from build123d import *

# Parameters (mm, degrees)
SKETCH2_R           = 3.175
SKETCH2_R_2         = 2
SKETCH2_R_3         = 1.905
SKETCH2_R_4         = 1.999999991
BOSS_EXTRUDE1_DEPTH = 6.35
FILLET3_R           = 2.54
FILLET4_R           = 2.54
FILLET5_R           = 2.54


with BuildPart() as part:
    # Sketch2 → Boss-Extrude1 (new body)
    with BuildSketch(Plane(origin=(0, 0, 0), x_dir=(1, 0, 0), z_dir=(0, 1, 0))):
        with BuildLine():
            Line((13.846627418, -27.11715969), (17.295902343, -28.359470371))
            Line((17.295902343, -28.359470371), (17.295902343, -164.950770806))
            Line((17.295902343, -164.950770806), (-5.788689103, -224.106088723))
            Line((-5.788689103, -224.106088723), (-16.51, -231.775))
            Line((-16.51, -231.775), (-16.51, -118.11))
            Line((-16.51, -118.11), (-16.51, -40.527182032))
            Line((-16.51, -40.527182032), (-12.5603, 0))
            ThreePointArc((-12.5603, 0), (0, 12.5603), (12.5603, 0))
            Line((12.5603, 0), (11.834308479, -23.392641285))
            ThreePointArc((11.834308479, -23.392641285), (12.129138804, -25.639224299), (13.846627418, -27.11715969))
        make_face()
        with Locations(Location((0, 0, 0), (0, 0, 270))):
            Circle(SKETCH2_R, mode=Mode.SUBTRACT)
        with Locations(Location((-11.43, -219.075, 0), (0, 0, 270))):
            Circle(SKETCH2_R_2, mode=Mode.SUBTRACT)
        with Locations(Location((-11.43, -212.725, 0), (0, 0, 270))):
            Circle(SKETCH2_R_2, mode=Mode.SUBTRACT)
        with Locations(Location((-11.43, -206.375, 0), (0, 0, 270))):
            Circle(SKETCH2_R_2, mode=Mode.SUBTRACT)
        with Locations(Location((-11.43, -200.025, 0), (0, 0, 270))):
            Circle(SKETCH2_R_2, mode=Mode.SUBTRACT)
        with Locations(Location((-10.6553, -63.5, 0), (0, 0, 270))):
            Circle(SKETCH2_R_3, mode=Mode.SUBTRACT)
        with Locations(Location((13.485902343, -38.1, 0), (0, 0, 270))):
            Circle(SKETCH2_R_4, mode=Mode.SUBTRACT)
        Polygon((-3.088444979, -200.025), (-8.437091633, -150.367410486), (11.707902343, -162.914359455), align=None, mode=Mode.SUBTRACT)
        Polygon((5.669829362, -152.570430441), (11.707902343, -156.331136136), (11.707902343, -148.173239335), align=None, mode=Mode.SUBTRACT)
        Polygon((-9.197164207, -143.310789567), (1.48362655, -149.963128939), (11.707902343, -142.517360277), (11.707902343, -83.82613362), (-6.752611098, -71.345410911), (-11.894481361, -75.089947663), (-11.894481361, -118.268516882), align=None, mode=Mode.SUBTRACT)
        with BuildLine():
            Line((-5.45038708, -57.047318199), (5.477174601, -46.119756518))
            Line((5.477174601, -46.119756518), (9.770631453, -46.119756518))
            Line((9.770631453, -46.119756518), (11.707902343, -77.037423395))
            Line((11.707902343, -77.037423395), (-4.240626345, -66.254995008))
            ThreePointArc((-4.240626345, -66.254995008), (-4.111536449, -61.554723114), (-5.45038708, -57.047318199))
        make_face(mode=Mode.SUBTRACT)
        Polygon((-10.6553, -40.527182032), (-8.00152211, -13.297230483), (5.477174601, -13.297230483), (5.477174601, -31.974105906), (1.94113758, -40.527182032), align=None, mode=Mode.SUBTRACT)
        Polygon((-10.6553, -44.022777243), (-10.6553, -51.472145687), (-0.991335505, -44.022777243), align=None, mode=Mode.SUBTRACT)
    extrude(amount=BOSS_EXTRUDE1_DEPTH)

    # Fillet3
    fillet3_edges = [part.edges().sort_by_distance(p)[0] for p in [
        (-5.788689103, 3.175, 224.106088723),
    ]]
    fillet(fillet3_edges, radius=FILLET3_R)

    # Fillet4
    fillet4_edges = [part.edges().sort_by_distance(p)[0] for p in [
        (-16.51, 3.175, 231.775),
    ]]
    fillet(fillet4_edges, radius=FILLET4_R)

    # Fillet5
    fillet5_edges = [part.edges().sort_by_distance(p)[0] for p in [
        (17.295902343, 3.175, 164.950770806),
    ]]
    fillet(fillet5_edges, radius=FILLET5_R)


solid = part.part
Build history of the part. All positions in model axes, mm. A direction names the side the tool comes from. Give positions to 0.01 mm unless a question says otherwise; leave off trailing zeros. Put each result on its own line as item: value.
Item 1: Pull direction Z, two halves, no side cores. Call faces 1 (the face through (12, 6.35, 107)), 2 (the face through (-12.2, 3.13, 201.87)), 3 (the face through (-0.276, 3.131, -12.557)): +Z half, -Z half, draft (parallel to the pull), parting line (faces both ways), or undercut.
Results are:
face 1: draft
face 2: undercut
face 3: -Z half
Item 2: Wall check: probe 1 along X at (y, z) = (4, 63.5); probe 2 along X at (y, z) = (0.5, 151.5); probe 3 along X at (y, z) = (0.75, 88). Give the ranges that are in metal, low to high.
Results are:
probe 1: -16.51 to -12.56, -8.75 to -3.98, 10.86 to 17.3
probe 2: -16.51 to -8.32, -6.62 to 7.14, 11.71 to 17.3
probe 3: -16.51 to -11.89, 11.71 to 17.3
Item 3: Cut at A-A on y = 2.75. Count the separate pieces of the cut face and the enclosed holes in it, then the cut area to 3 significant figures.
Results are:
separate pieces: 1
enclosed holes: 13
area: 4,000 mm2
Item 4: Which spindle directions (+Z, -Z, +X, -X, +Y, -Y) get a long thin tool onto all of the face, cutting with end or side? Do faces 4 (the face through (2.607, 3.131, 77.673)), 5 (the face through (-14.563, 3.131, 20.547)). Say none if no direction does.
Results are:
face 4: +Y, -Y
face 5: -Z, -X, +Y, -Y
Item 5: Drop flat-ended pins along their axis: pin 1 Ø3 at (y, z) = (2.5, 23) entering from -X; pin 2 Ø3 at (x, y) = (2.5, 1.5) entering from -Z. Give the stop position or say it passes through.
Results are:
pin 1: x = -14.95
pin 2: z = -12.52
